Check sheet for the modelled part. Datum: model origin and axes. Units: mm. Face numbers are marked on the shaded views. A direction names the side the tool comes from. Give positions to 0.01 mm unless a question says otherwise; leave off trailing zeros. Write each loop counter-clockwise with the first axis right and the second up, starting at its lowest first coordinate (ties: lowest second). Pieces come first, ordered by that corner, then holes. Notation, with made-up numbers: M 84.5,44 L 129.5,44 A21 ccw 129.5,65 Z; hole C -17,6 d4. An arc over 180 degrees is marked long. Write each question's results on one line, items separated by ' | '. Start each with the question number.
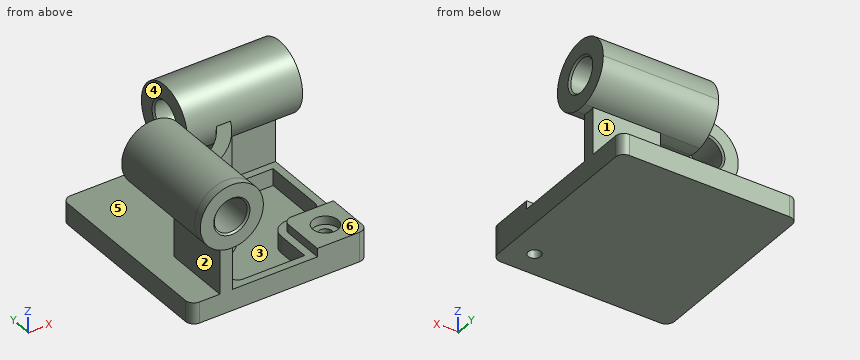
from build123d import *

# Parameters (mm, degrees)
F0_W            = 210
F0_H            = 225
F1_DEPTH        = 25
F3_DEPTH        = 95
F4_R            = 37.5
F5_DEPTH        = 10
F5_DEPTH_BACK   = 127
F7_DEPTH        = 10
F7_DEPTH_BACK   = 127
F8_W            = 60
F8_H            = 60
F9_DEPTH        = 10
F10_R           = 10
F12_DEPTH       = 20
F14_D           = 15
F14_CBORE_D     = 30
F14_CBORE_DEPTH = 10
F15_R           = 10
F17_R           = 19.5
F18_DEPTH       = 220.001
F16_R           = 19.5
F19_DEPTH       = 235.001
F20_SIZE        = 2
F21_R           = 10


with BuildPart() as f1:
    # F0 (on Top) → F1 (new body)
    with BuildSketch(Plane.XY):
        with Locations((-36.6346123987, -2.6086959988)):
            Rectangle(F0_W, F0_H)
    extrude(amount=F1_DEPTH)

    # F2 (on face) → F3 (join)
    with BuildSketch(Plane.XY.offset(25)):
        with BuildLine():
            Line((68.3653876013, 45.8913040012), (68.3653876013, 60.8913040012))
            Line((68.3653876013, 60.8913040012), (-11.6346123987, 60.8913040012))
            ThreePointArc((-11.6346123987, 60.8913040012), (-39.7523614048, -6.9909469927), (-107.6346123987, -35.1086959988))
            Line((-107.6346123987, -35.1086959988), (-107.6346123987, -115.1086959988))
            Line((-107.6346123987, -115.1086959988), (-92.6346123987, -115.1086959988))
            Line((-92.6346123987, -115.1086959988), (-92.6346123987, -49.0905126777))
            ThreePointArc((-92.6346123987, -49.0905126777), (-29.145759687, -17.5975487105), (2.3472042802, 45.8913040012))
            Line((2.3472042802, 45.8913040012), (68.3653876013, 45.8913040012))
        make_face()
    extrude(amount=F3_DEPTH)

    # F4 (on face) → F5 (join, two sides)
    with BuildSketch(Plane.XZ.offset(115.1086959988)) as f5_sk:
        with Locations((-100.1346123987, 120)):
            Circle(F4_R)
    extrude(amount=F5_DEPTH)
    extrude(f5_sk.sketch, amount=-F5_DEPTH_BACK)

    # F6 (on face) → F7 (join, two sides)
    with BuildSketch(Plane.YZ.offset(68.3653876013)) as f7_sk:
        with BuildLine():
            ThreePointArc((60.8913040012, 80.7094158862), (84.2133740161, 94.504902432), (93.3913040012, 120))
            ThreePointArc((93.3913040012, 120), (27.8962064332, 150.8220700148), (45.8913040012, 80.7094158862))
            Line((45.8913040012, 80.7094158862), (45.8913040012, 120))
            Line((45.8913040012, 120), (60.8913040012, 120))
            Line((60.8913040012, 120), (60.8913040012, 80.7094158862))
        make_face()
        with BuildLine():
            Line((45.8913040012, 120), (45.8913040012, 80.7094158862))
            ThreePointArc((45.8913040012, 80.7094158862), (53.3913040012, 80), (60.8913040012, 80.7094158862))
            Line((60.8913040012, 80.7094158862), (60.8913040012, 120))
            Line((60.8913040012, 120), (45.8913040012, 120))
        make_face()
    extrude(amount=F7_DEPTH)
    extrude(f7_sk.sketch, amount=-F7_DEPTH_BACK)

    # F8 (on face) → F9 (join)
    with BuildSketch(Plane.XY.offset(25)):
        with Locations((38.3653876013, -85.1086959988)):
            Rectangle(F8_W, F8_H)
    extrude(amount=F9_DEPTH)

    # F10
    f10_edges = [f1.edges().sort_by_distance(p)[0] for p in [
        (8.365388, -55.108696, 30),
    ]]
    fillet(f10_edges, radius=F10_R)

    # F11 (on face) → F12 (cut)
    with BuildSketch(Plane.XY.offset(25)):
        with BuildLine():
            ThreePointArc((9.9408952549, 36.8913040012), (-22.7817986563, -23.9615097412), (-83.6346123987, -56.6842036524))
            Line((-83.6346123987, -56.6842036524), (-83.6346123987, -106.1086959988))
            Line((-83.6346123987, -106.1086959988), (-0.6346123987, -106.1086959988))
            Line((-0.6346123987, -106.1086959988), (-0.6346123987, -65.1086959988))
            ThreePointArc((-0.6346123987, -65.1086959988), (4.9303587587, -51.6736671562), (18.3653876013, -46.1086959988))
            Line((18.3653876013, -46.1086959988), (59.3653876013, -46.1086959988))
            Line((59.3653876013, -46.1086959988), (59.3653876013, 36.8913040012))
            Line((59.3653876013, 36.8913040012), (9.9408952549, 36.8913040012))
        make_face()
    extrude(amount=-F12_DEPTH, mode=Mode.SUBTRACT)

    # F14 (through all)
    with Locations(Plane.XY.offset(35)):
        with Locations((38.3653876013, -85.1086959988)):
            CounterBoreHole(F14_D / 2, F14_CBORE_D / 2, F14_CBORE_DEPTH)

    # F15
    f15_edges = [f1.edges().sort_by_distance(p)[0] for p in [
        (-83.634612, -56.684204, 15),
        (9.940895, 36.891304, 15),
        (-83.634612, -106.108696, 15),
        (59.365388, -46.108696, 15),
    ]]
    fillet(f15_edges, radius=F15_R)

    # F17 (on face) → F18 (cut, through all)
    with BuildSketch(Plane.YZ.offset(78.3653876013)):
        with Locations((53.3913040012, 120)):
            Circle(F17_R)
    extrude(amount=-F18_DEPTH, mode=Mode.SUBTRACT)

    # F16 (on face) → F19 (cut, through all)
    with BuildSketch(Plane.XZ.offset(125.1086959988)):
        with Locations((-100.1346123987, 120)):
            Circle(F16_R)
    extrude(amount=-F19_DEPTH, mode=Mode.SUBTRACT)

    # F20
    f20_edges = [f1.edges().sort_by_distance(p)[0] for p in [
        (-119.634612, -125.108696, 120),
        (78.365388, 33.891304, 120),
        (-119.634612, 11.891304, 120),
        (-58.634612, 33.891304, 120),
    ]]
    chamfer(f20_edges, length=F20_SIZE)

    # F21
    f21_edges = [f1.edges().sort_by_distance(p)[0] for p in [
        (68.365388, -115.108696, 17.5),
        (-141.634612, -115.108696, 12.5),
        (68.365388, 109.891304, 12.5),
        (-141.634612, 109.891304, 12.5),
    ]]
    fillet(f21_edges, radius=F21_R)


solid = f1.part
Q1. Depth check by flat-ended pin: pin 1 Ø1 at (x, z) = (-76, 50.5) entering from -Y; pin 2 Ø3 at (x, y) = (-29.5, 0) entering from +Z; pin 3 Ø10 at (x, z) = (-116.5, 80.5) entering from -Y; pin 4 Ø3 at (x, z) = (37.5, 32.5) entering from +Y. Enter the tip coordinate at first touch or a pass-through.
Q2. Scan lines: L1, parallel to X at y = -101.5, z = 118.5; L2, parallel to Z at x = -113, y = -8.5; L3, parallel to Z at x = 28, y = -75. Record each from-to range of solid material in increasing order.
Q3. Release check for a two-part mould opening along X. For the marked faces 1, 2 and 3 record: pulls with the +X half, pulls with the -X half, needs draft (parallel to the pull), parting line crosses it, or undercut.
Q4. Tool access check on the marked faces 4, 5 and 6. Record the directions out of +Z, -Z, +X, -X, +Y, -Y that give a thin tool (end or side, any length) a straight path to the whole face; none if there is none.
Q5. Section check C-C on z = 145.5. Record the boundary of the cut face in (x, y).
Q6. Section check B-B on x = 40. Record the boundary of the cut face in (y, z).
Q7. Section check D-D on z = 14. Record the boundary of the cut face in (x, y), plus the area to 3 significant figures.
Q8. Section check A-A on z = 68.5. Record the boundary of the cut face in (x, y), plus the area to 3 significant figures.
Check result:
1) pin 1: y = -45.65 | pin 2: z = 120 | pin 3: through | pin 4: y = 60.89
2) L1: -137.6 to -119.58, -80.69 to -62.66 | L2: 0 to 25, 84.78 to 105.35, 134.65 to 155.22 | L3: 0 to 25
3) face 1: needs draft | face 2: pulls with the -X half | face 3: undercut
4) face 4: +Z, -X, +Y | face 5: -X, +Y | face 6: +Z, +X, -Y
5) outline: M -127.63,-125.11 L -72.64,-125.11 L -72.64,11.89 L -127.63,11.89 Z; M -58.63,22.57 L 78.37,22.57 L 78.37,84.21 L -58.63,84.21 Z
6) outline: M -115.11,0 L -92.43,0 L -92.43,25 L -100.02,25 L -100.02,35 L -115.11,35 Z; M -77.79,0 L 109.89,0 L 109.89,25 L 60.89,25 L 60.89,80.71 A40 ccw long 45.89,80.71 L 45.89,25 L 36.89,25 L 36.89,5 L -46.11,5 L -46.11,25 L -55.11,25 L -55.11,35 L -70.2,35 L -70.2,25 L -77.79,25 Z; hole C 53.39,120 d39
7) outline: M -141.63,-105.11 A10 ccw -131.63,-115.11 L 58.37,-115.11 A10 ccw 68.37,-105.11 L 68.37,99.89 A10 ccw 58.37,109.89 L -131.63,109.89 A10 ccw -141.63,99.89 Z; hole M -83.63,-96.11 A10 ccw -73.63,-106.11 L -0.63,-106.11 L -0.63,-65.11 A19 cw 18.37,-46.11 L 49.37,-46.11 A10 ccw 59.37,-36.11 L 59.37,36.89 L 17.84,36.89 A10 ccw 8.19,29.51 A120 cw -76.25,-54.93 A10 ccw -83.63,-64.58 Z; hole C 38.37,-85.11 d15 | area: 36,300 mm^2
8) outline: M -107.63,-115.11 L -92.63,-115.11 L -92.63,-49.09 A111 ccw 2.35,45.89 L 68.37,45.89 L 68.37,60.89 L -11.63,60.89 A96 cw -107.63,-35.11 Z | area: 4,400 mm^2
